Source: CAD feature listing. Evaluate the final solid. Frame: model axes, mm. A direction names the side the tool comes from. Coordinates: 2 decimals unless noted, no trailing zeros. Write each loop counter-clockwise with the first axis right and the second up, starting at its lowest first coordinate (ties: lowest second). Pieces come first, ordered by that corner, then holes. Notation, with made-up numbers: (70.25, -4) - (129.25, -4) arc R9 ccw to (129.25, 8) - close; hole circle Ø6 at (52, -7). An arc over 180 degrees is marked (long way). One line per question, with ' | ' between items.
from build123d import *

# Parameters (mm, degrees)
SKETCH005_W     = 48.896005
SKETCH005_H     = 53.655467
PAD003_DEPTH    = 1
SKETCH006_W     = 46.796005
SKETCH006_H     = 51.555467
PAD004_DEPTH    = 2
SKETCH007_R     = 0.95
SKETCH007_R_2   = 1.001433
SKETCH007_R_3   = 1
SKETCH007_R_4   = 0.951025
PAD005_DEPTH    = 3
SKETCH008_R     = 2.5
POCKET002_DEPTH = 2
SKETCH009_R     = 1.5
POCKET003_DEPTH = 5
SKETCH010_W     = 7.035641
SKETCH010_H     = 2
SKETCH010_W_2   = 7.054697
SKETCH010_W_3   = 7.079575
POCKET004_DEPTH = 1
SKETCH011_R     = 2
POCKET005_DEPTH = 5


with BuildPart() as part:
    # Sketch005 (on Face1 of CopyBinder) → Pad003 (new body)
    with BuildSketch(Plane.XY.offset(6.0393)):
        with Locations((23.137507, 25.410293)):
            Rectangle(SKETCH005_W, SKETCH005_H)
    extrude(amount=PAD003_DEPTH)

    # Sketch006 (on Face5 of Pad003) → Pad004 (join)
    with BuildSketch(Plane(origin=(0, 0, 6.0393), x_dir=(1, 0, 0), z_dir=(0, 0, -1))):
        with Locations((23.137507, -25.410293)):
            Rectangle(SKETCH006_W, SKETCH006_H)
    extrude(amount=PAD004_DEPTH)

    # Sketch007 (on Face2 of Binder001) → Pad005 (join)
    with BuildSketch(Plane.XY.offset(1.0393)):
        with Locations((4.794625, 2.000882)):
            Circle(SKETCH007_R)
        with Locations((16.190751, 1.997755)):
            Circle(SKETCH007_R_2)
        with Locations((27.124204, 11.274795)):
            Circle(SKETCH007_R_3)
        with Locations((27.14775, 36.64242)):
            Circle(SKETCH007_R_3)
        with Locations((16.21209, 49.004375)):
            Circle(SKETCH007_R_4)
        with Locations((4.787556, 48.988897)):
            Circle(SKETCH007_R)
    extrude(amount=PAD005_DEPTH)

    # Sketch008 (on Face5 of Pad005) → Pocket002 (cut)
    with BuildSketch(Plane.XY.offset(7.0393)):
        with Locations((27.08551, 47.738026)):
            Circle(SKETCH008_R)
        with Locations((27.08551, 3.082559)):
            Circle(SKETCH008_R)
    extrude(amount=-POCKET002_DEPTH, mode=Mode.SUBTRACT)

    # Sketch009 (on Face14 of Pocket002) → Pocket003 (cut)
    with BuildSketch(Plane.XY.offset(5.0393)):
        with Locations((27.08551, 3.082559)):
            Circle(SKETCH009_R)
        with Locations((27.08551, 47.738026)):
            Circle(SKETCH009_R)
    extrude(amount=-POCKET003_DEPTH, mode=Mode.SUBTRACT)

    # Sketch010 (on Face8 of Pocket003) → Pocket004 (cut)
    with BuildSketch(Plane.YZ.offset(46.53551)):
        with Locations((23.944557, 5.0393)):
            Rectangle(SKETCH010_W, SKETCH010_H)
        with Locations((34.439561, 5.0393)):
            Rectangle(SKETCH010_W_2, SKETCH010_H)
        with Locations((13.454822, 5.0393)):
            Rectangle(SKETCH010_W_3, SKETCH010_H)
    extrude(amount=-POCKET004_DEPTH, mode=Mode.SUBTRACT)

    # Sketch011 (on Face4 of Pocket004) → Pocket005 (cut)
    with BuildSketch(Plane.XY.offset(7.0393)):
        with Locations((6.969133, 38.932186)):
            Circle(SKETCH011_R)
    extrude(amount=-POCKET005_DEPTH, mode=Mode.SUBTRACT)


solid = part.part
Item 1: Mould query, pull axis X, two halves, no side actions, for faces 4 (the face through (4.66, 49.93, 2.52)), 5 (the face through (5, 2, 1.039)), 6 (the face through (46.536, 29, 5)). Classes: pulls with the +X half, pulls with the -X half, needs draft (parallel to the pull), parting line crosses it, or undercut.
Check sheet entries:
face 4: undercut | face 5: needs draft | face 6: pulls with the +X half
Item 2: Cut plane D-D on z = 3.4. Return loops of the section in (x, y), and give its area (3 significant figures).
Check sheet entries:
outline: circle Ø1.9 at (4.79, 2); circle Ø1.9 at (4.79, 48.99); circle Ø2 at (16.19, 2); circle Ø1.9 at (16.21, 49); circle Ø2 at (27.12, 11.27); circle Ø2 at (27.15, 36.64) | area: 17.9 mm²
Item 3: Cut plane A-A on x = 27. State how many separate pieces and enclosed holes the cut face has, and give its area (3 significant figures).
Check sheet entries:
separate pieces: 3 | enclosed holes: 0 | area: 143 mm²
Item 4: Cut plane B-B on y = 47. Return loops of the section in (x, z).
Check sheet entries:
outline: (-1.31, 6.04) - (-0.26, 6.04) - (-0.26, 4.04) - (25.78, 4.04) - (25.78, 5.04) - (24.7, 5.04) - (24.7, 7.04) - (-1.31, 7.04) - close; (28.39, 4.04) - (46.54, 4.04) - (46.54, 6.04) - (47.59, 6.04) - (47.59, 7.04) - (29.47, 7.04) - (29.47, 5.04) - (28.39, 5.04) - close
Item 5: Pin query (flat end, axial travel): pin 1 Ø0.5 at (x, z) = (46, 4.5) entering from +Y; pin 2 Ø1.8 at (x, y) = (27.09, 47.74) entering from +Z; pin 3 Ø3 at (y, z) = (36, 2) entering from +X; pin 4 Ø0.5 at (x, z) = (46, 5) entering from -Y. Return the tip coordinate at first contact, or that it passes through.
Check sheet entries:
pin 1: y = 51.19 | pin 2: through | pin 3: x = 28.15 | pin 4: y = -0.37
Item 6: Access query for faces 1 (the face through (45.536, 24, 5)), 2 (the face through (29.395, 46.781, 6.053)), 3 (the face through (15.511, 49.647, 2.518)). Directions: +Z, -Z, +X, -X, +Y, -Y. A direction counts if a zero-diameter tool reaches every point of the face in a straight line with its end or side. Return the directions, or none.
Check sheet entries:
face 1: -Z, +X | face 2: +Z | face 3: -Z
Item 7: Ray query, line 1 along X through (y, z) = (49, 2.75); line 2 along X through (y, z) = (29.5, 5.7); line 3 along Z through (x, y) = (6, 48). Return the intervals inside material, ascending. Write a range as [from, to].
Check sheet entries:
line 1: [3.84, 5.74], [15.26, 17.16] | line 2: [-0.26, 46.54] | line 3: [4.04, 7.04]
Item 8: Cut plane C-C on x = 37. Return loops of the section in (y, z).
Check sheet entries:
outline: (-1.42, 6.04) - (-0.37, 6.04) - (-0.37, 4.04) - (51.19, 4.04) - (51.19, 6.04) - (52.24, 6.04) - (52.24, 7.04) - (-1.42, 7.04) - close
